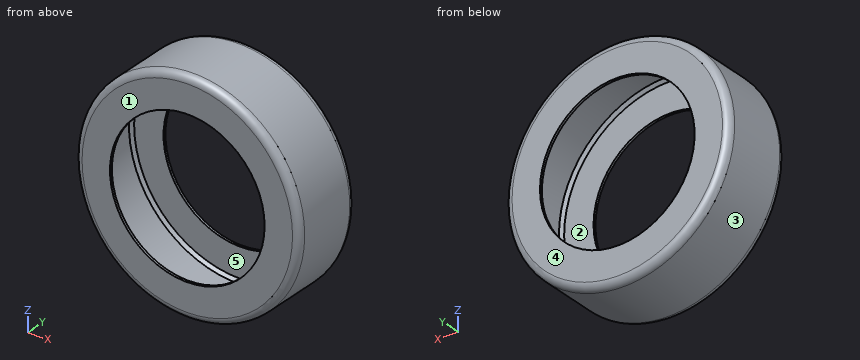
from build123d import *

# Parameters (mm, degrees)
FILLET2_R     = 0.7
CHAMFER1_SIZE = 0.3


with BuildPart() as part:
    # Sketch1 → Revolve1 (revolve)
    with BuildSketch(Plane.XY, mode=Mode.PRIVATE) as revolve1_sk:
        Polygon((-11.25, 3.75), (-11.25, -3.75), (-7.75, -3.75), (-7.75, -3.5), (-11, -3.5), (-11, 3.5), (-7.75, 3.5), (-7.75, 3.75), align=None)
    revolve(revolve1_sk.sketch.rotate(Axis((0, -3.75, 0), (0, 1, 0)), 180), axis=Axis((0, -3.75, 0), (0, 1, 0)))

    # Fillet2
    fillet2_edges = [part.edges().sort_by_distance(p)[0] for p in [
        (-11.25, 3.75, 0),
        (-11.25, -3.75, 0),
    ]]
    fillet(fillet2_edges, radius=FILLET2_R)

    # Chamfer1
    chamfer1_edges = [part.edges().sort_by_distance(p)[0] for p in [
        (-11, -3.5, 0),
        (-11, 3.5, 0),
    ]]
    chamfer(chamfer1_edges, length=CHAMFER1_SIZE)


solid = part.part
Could you check a few things on this model? Use its own coordinates, in mm. Face numbers are marked on the shaded views. A direction names the side the tool comes from. Coordinates: 2 decimals unless noted, no trailing zeros. Order: outer loops, then holes, each group sorted by start corner. A loop starts at its lowest first (then second) coordinate and runs counter-clockwise, first axis right, second up. Notation, with made-up numbers: (80.25, 35.5) -> (136.25, 35.5) arc R4 ccw to (136.25, 39.5) -> close; hole circle Ø11 at (38.5, -18.75). An arc over 180 degrees is marked (long way). One line per item, written item: value. Start each with the question number.
1) Which directions (+Z, -Z, +X, -X, +Y, -Y) give clear straight access to the entire face, cutting with the end or side of a thin tool? Please do the marked faces 4 and 5.
2) If I drill on L1, parallel to Y at x = -8, z = 3; L2, parallel to Z at x = 0.25, y = 0.75; L3, parallel to X at y = -1.5, z = 8.75, over which ranges is the centre line in solid material (lowest first)? Write a range as [from, to].
3) Imagine slicing it at A-A on z = 0. List the corners of the cut face in (x, y) for me.
4) Imagine slicing it at B-B on x = 0. List the corners of the cut face in (y, z) for me, plus the area to 3 significant figures.
5) I'm going to push flat-ended pins straight in: pin 1 (4 mm diameter, centred on y = -0.5, z = 6, fed in from +X); pin 2 (2 mm diameter, centred on x = -5, y = 1.5, fed in from -Z); pin 3 (3 mm diameter, centred on x = -5, y = 2.5, fed in from +Z). Where does each tip first touch, or does it pass through?
6) We'd pull the mould along Y, two halves only. Please class the marked faces 1, 2 and 3: +Y half, -Y half, draft (parallel to the pull), parting line (faces both ways), or undercut.
7) Imagine slicing it at C-C on y = -1.5. List the corners of the cut face in (x, z) for me.
Answer list:
1. face 4: +Z, -Z, +X, -X, +Y
1. face 5: none
2. L1: y = [-3.75, -3.5], [3.5, 3.75]
2. L2: z = [-11.25, -11], [11, 11.25]
2. L3: x = [-7.07, -6.67], [6.67, 7.07]
3. outline: (-11.25, -3.05) arc R0.7 ccw to (-10.55, -3.75) -> (-7.75, -3.75) -> (-7.75, -3.5) -> (-10.7, -3.5) -> (-11, -3.2) -> (-11, 3.2) -> (-10.7, 3.5) -> (-7.75, 3.5) -> (-7.75, 3.75) -> (-10.55, 3.75) arc R0.7 ccw to (-11.25, 3.05) -> close; (7.75, -3.75) -> (10.55, -3.75) arc R0.7 ccw to (11.25, -3.05) -> (11.25, 3.05) arc R0.7 ccw to (10.55, 3.75) -> (7.75, 3.75) -> (7.75, 3.5) -> (10.7, 3.5) -> (11, 3.2) -> (11, -3.2) -> (10.7, -3.5) -> (7.75, -3.5) -> close
4. outline: (-3.75, -10.55) arc R0.7 ccw to (-3.05, -11.25) -> (3.05, -11.25) arc R0.7 ccw to (3.75, -10.55) -> (3.75, -7.75) -> (3.5, -7.75) -> (3.5, -10.7) -> (3.2, -11) -> (-3.2, -11) -> (-3.5, -10.7) -> (-3.5, -7.75) -> (-3.75, -7.75) -> close; (-3.75, 7.75) -> (-3.5, 7.75) -> (-3.5, 10.7) -> (-3.2, 11) -> (3.2, 11) -> (3.5, 10.7) -> (3.5, 7.75) -> (3.75, 7.75) -> (3.75, 10.55) arc R0.7 ccw to (3.05, 11.25) -> (-3.05, 11.25) arc R0.7 ccw to (-3.75, 10.55) -> close
4. area: 6.76 mm2
5. pin 1: stops at x = 10.51
5. pin 2: stops at z = -10.51
5. pin 3: stops at z = 10.69
6. face 1: -Y half
6. face 2: undercut
6. face 3: draft
7. outline: circle Ø22.5 at (0, 0); hole circle Ø22 at (0, 0)
